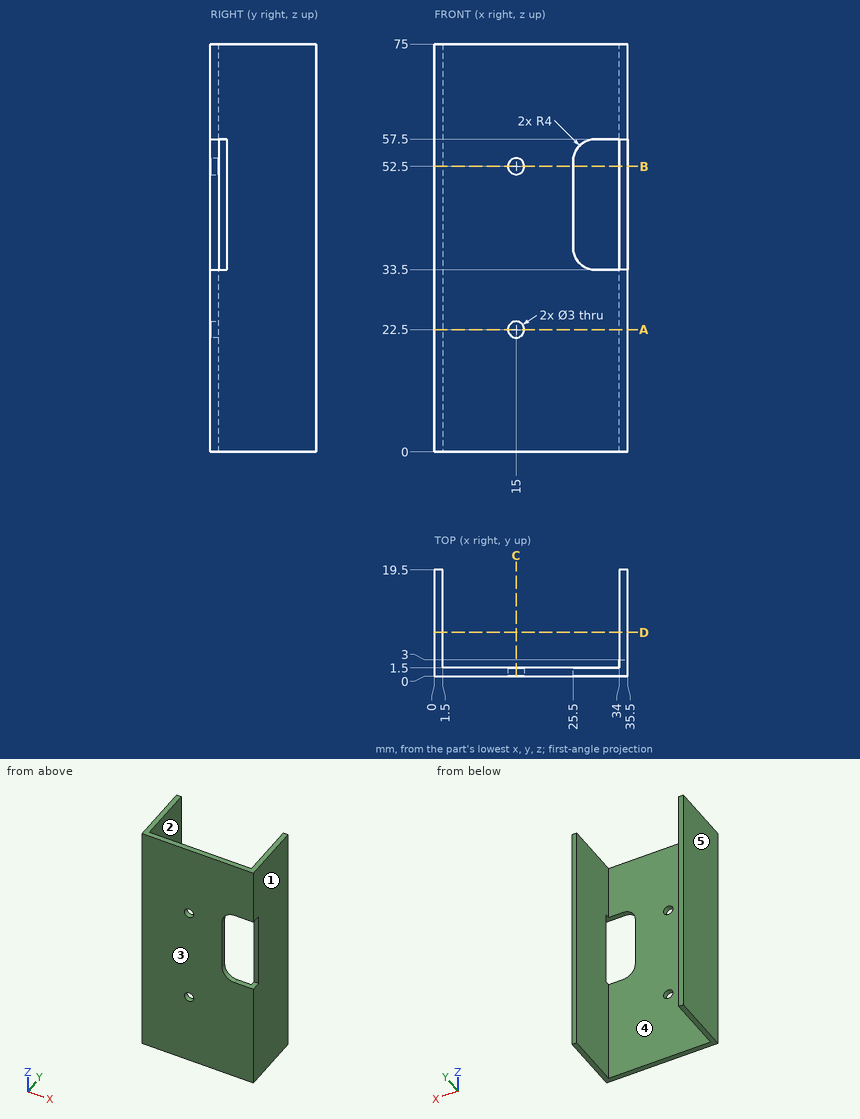
Design review of the part shown in the three views and the two pictorial views. Dimensions are in mm from the part's minimum x, y and z. A direction names the side the tool comes from. Round coordinates to 2 decimals unless told otherwise and drop trailing zeros. Loops run counter-clockwise (first coordinate to the right, second up) from the corner with the lowest first, then second, coordinate; pieces in that order, holes last.
(1) We need section C-C (x = 15). Give the boundary of the cut face in (y, z).
Returned:
outline: (0, 0) - (1.5, 0) - (1.5, 21) - (0, 21) - close; (0, 24) - (1.5, 24) - (1.5, 51) - (0, 51) - close; (0, 54) - (1.5, 54) - (1.5, 75) - (0, 75) - close
(2) Tool access review of the marked faces 1 and 2: name each direction out of +Z, -Z, +X, -X, +Y, -Y from which nothing blocks a thin tool from reaching the whole face with its end or side.
Returned:
face 1: +Z, -Z, +X, +Y, -Y
face 2: +Z, -Z, +Y
(3) We need section A-A (z = 22.5). Give the boundary of the cut face in (x, y).
Returned:
outline: (0, 0) - (13.5, 0) - (13.5, 1.5) - (1.5, 1.5) - (1.5, 19.5) - (0, 19.5) - close; (16.5, 0) - (35.5, 0) - (35.5, 19.5) - (34, 19.5) - (34, 1.5) - (16.5, 1.5) - close
(4) Wall thickness on line 1 along X through (y, z) = (0.4, 22.5); line 2 along X through (y, z) = (3.25, 36); line 3 along Y through (x, z) = (18.5, 32): over which ranges is each line inside the solid? List them lowest first.
Returned:
line 1: x = 0 to 13.5, 16.5 to 35.5
line 2: x = 0 to 1.5, 34 to 35.5
line 3: y = 0 to 1.5
(5) We need section D-D (y = 8). Give the boundary of the cut face in (x, z).
Returned:
outline: (0, 0) - (1.5, 0) - (1.5, 75) - (0, 75) - close; (34, 0) - (35.5, 0) - (35.5, 75) - (34, 75) - close
(6) We need section B-B (z = 52.5). Give the boundary of the cut face in (x, y).
Returned:
outline: (0, 0) - (13.5, 0) - (13.5, 1.5) - (1.5, 1.5) - (1.5, 19.5) - (0, 19.5) - close; (16.5, 0) - (25.5, 0) - (25.5, 1.5) - (16.5, 1.5) - close; (34, 3) - (35.5, 3) - (35.5, 19.5) - (34, 19.5) - close
(7) Mouldability with a two-part tool opening along X and no side actions: class the marked faces 3, 4 and 5 as released by +X, released by -X, zero draft, split by the parting line, or undercut.
Returned:
face 3: zero draft
face 4: undercut
face 5: released by -X
(8) Clearance check with flat-ended pins moving along their axes: P1, Ø2.5, axis at x = 15, z = 22.5, coming from the -Y side; P2, Ø1.6, axis at x = 34.5, z = 50.5, coming from the -Y side; P3, Ø0.8, axis at y = 0.5, z = 41.5, coming from the +X side; P4, Ø4, axis at x = 15, z = 52.5, coming from the +Y side. State where each tip first meets the part, or that it passes through.
Returned:
P1: passes through
P2: stops at y = 3
P3: stops at x = 25.5
P4: stops at y = 1.5
